from build123d import *

# Parameters (mm, degrees)
F1_DEPTH = 1000


with BuildPart() as f1:
    # F0 (on Front) → F1 (new body)
    with BuildSketch(Plane.XZ):
        with BuildLine():
            Line((50, -50), (50, -40))
            Line((50, -40), (15, -40))
            ThreePointArc((15, -40), (6.514719, -36.485281), (3, -28))
            Line((3, -28), (3, 0))
            Line((3, 0), (3, 28))
            ThreePointArc((3, 28), (6.514719, 36.485281), (15, 40))
            Line((15, 40), (50, 40))
            Line((50, 40), (50, 50))
            Line((50, 50), (0, 50))
            Line((0, 50), (-50, 50))
            Line((-50, 50), (-50, 40))
            Line((-50, 40), (-15, 40))
            ThreePointArc((-15, 40), (-6.514719, 36.485281), (-3, 28))
            Line((-3, 28), (-3, 0))
            Line((-3, 0), (-3, -28))
            ThreePointArc((-3, -28), (-6.514719, -36.485281), (-15, -40))
            Line((-15, -40), (-50, -40))
            Line((-50, -40), (-50, -50))
            Line((-50, -50), (0, -50))
            Line((0, -50), (50, -50))
        make_face()
    extrude(amount=-F1_DEPTH)


solid = f1.part
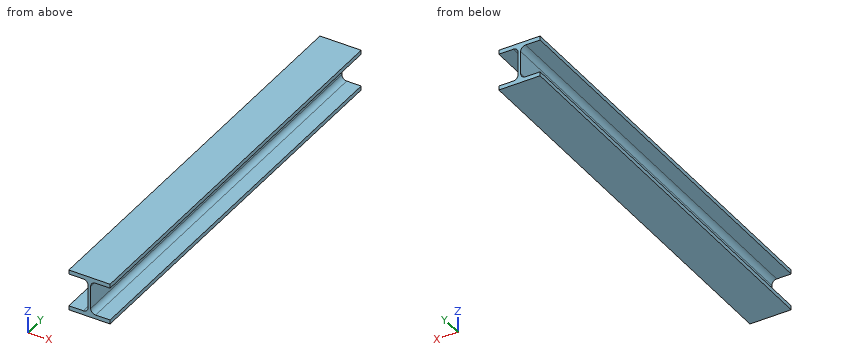
Could you check a few things on this model? Use its own coordinates, in mm. Give positions to 0.01 mm unless a question says otherwise; leave off trailing zeros. Loops run counter-clockwise (first coordinate to the right, second up) from the corner with the lowest first, then second, coordinate; pieces in that order, holes last. Notation, with made-up numbers: (-36, 69) -> (7, 69) arc R18 ccw to (7, 96) -> close; hole circle Ø9 at (-17.5, 87.25). An arc over 180 degrees is marked (long way). Answer as CSV lines item,"result". Start each with the question number.
(1) If we section it at A-A on x = 36.5: Write out the boundary of the cut face in (y, z).
(2) If we section it at B-B on y = 505: Write out the boundary of the cut face in (x, z), then the cut area to 3 significant figures.
(3) I'm going to push flat-ended pins straight in: pin 1 Ø4 at (y, z) = (781, 18.5) entering from +X; pin 2 Ø6 at (y, z) = (559, -21) entering from -X. Where does each tip first touch, or does it pass through?
(4) If we section it at C-C on z = -8: Write out the boundary of the cut face in (x, y).
(5) I need wall thicknesses on probe 1 along Z at (x, y) = (-26, 140); probe 2 along X at (y, z) = (491, -23.5); probe 3 along Z at (x, y) = (11, 408.5). Which ranges of each line are inside material? Lowest first, please.
Computed:
1,outline,"(0, -50) -> (1000, -50) -> (1000, -40) -> (0, -40) -> close; (0, 40) -> (1000, 40) -> (1000, 50) -> (0, 50) -> close"
2,outline,"(-50, -50) -> (50, -50) -> (50, -40) -> (15, -40) arc R12 cw to (3, -28) -> (3, 28) arc R12 cw to (15, 40) -> (50, 40) -> (50, 50) -> (-50, 50) -> (-50, 40) -> (-15, 40) arc R12 cw to (-3, 28) -> (-3, -28) arc R12 cw to (-15, -40) -> (-50, -40) -> close"
2,area,"2,600 mm2"
3,pin 1,"stops at x = 3"
3,pin 2,"stops at x = -3"
4,outline,"(-3, 0) -> (3, 0) -> (3, 1000) -> (-3, 1000) -> close"
5,probe 1,"z = -50 to -40, 40 to 50"
5,probe 2,"x = -3 to 3"
5,probe 3,"z = -50 to -39.31, 39.31 to 50"
